```python
from build123d import *

# Parameters (mm, degrees)
SKETCH2_R = 12.85


with BuildPart() as part:
    # Sweep1: sweep along a path in Sketch1
    with BuildLine() as sweep1_path:  # in the path sketch's own coordinates; laid on its plane below (add() does not lay a ready-made edge on the line's plane)
        Line((301.307150881, 29.86530187), (131.307150881, 29.86530187))
        add(Edge.make_bspline(
            [(131.307150881, 29.86530187), (90.533603326, 8.116674685), (47, 8.116674685)],
            knots=[0, 0, 0, 1, 1, 1], degree=2))
        Line((47, 8.116674685), (0, 8.116674685))
    # Sketch2 → Sweep1 (sweep)
    with BuildSketch(Plane(origin=(301.307150881, 0, 0), x_dir=(0, 0, -1), z_dir=(1, 0, 0))):
        with Locations((29.86530187, 0)):
            Circle(SKETCH2_R)
    sweep1 = sweep(path=Plane(origin=(0, 0, 0), x_dir=(1, 0, 0), z_dir=(0, 1, 0)) * sweep1_path.line, transition=Transition.RIGHT)

    # Mirror1: Sweep1 across plane
    add(sweep1.mirror(Plane(origin=(0, 0, 0), x_dir=(0, 0, 1), z_dir=(1, 0, 0))))


solid = part.part
```
Source: CAD feature listing. Evaluate the final solid. Frame: model axes, mm. A direction names the side the tool comes from. Coordinates: 2 decimals unless noted, no trailing zeros. Loops run counter-clockwise (first coordinate to the right, second up) from the corner with the lowest first, then second, coordinate; pieces in that order, holes last. Notation, with made-up numbers: (-23.5, 11.25) - (26.5, 11.25) arc R10 cw to (26.5, 23.25) - close; hole circle Ø4 at (72, -7). An arc over 180 degrees is marked (long way). Answer as CSV lines item,"result".
1. Mould query, pull axis X, two halves, no side actions, for faces 1 (the cylindrical face through (-213.488, 4.922, -41.735)), 2 (the flat face through (-301.307, 0, -30)), 3 (the cylindrical face through (0.658, 4.922, -19.987)). Classes: released by +X, released by -X, zero draft, split by the parting line, or undercut.
Established:
face 1,"zero draft"
face 2,"released by -X"
face 3,"undercut"
2. Reachability of faces 4 (the flat face through (301.307, 0, -30)), 5 (the cylindrical face through (213.488, 4.922, -41.735)) from +Z, -Z, +X, -X, +Y, -Y: full face, straight path, thin tool, end or side. Return the list, or none.
Established:
face 4,"+Z, -Z, +X, +Y, -Y"
face 5,"+X"
3. Contact query for flat-ended pins moving along their axis: pin 1 (5 mm diameter, centred on x = 38.5, z = -19.5, fed in from +Y); pin 2 (10 mm diameter, centred on x = -78.5, y = -3.5, fed in from -Z); pin 3 (3 mm diameter, centred on x = -143, z = -18.5, fed in from +Y). Output: stop coordinate, or through.
Established:
pin 1,"stops at y = 9.28"
pin 2,"stops at z = -25.03"
pin 3,"stops at y = 8.23"
4. Ray query, line 1 (X direction, y = -4.25, z = -35.5); line 2 (Z direction, x = 4, y = -1.75); line 3 (Y direction, x = 73, z = -10.5). Return the intervals inside material, ascending.
Established:
line 1,"x = -301.31 to -115.38, 115.38 to 301.31"
line 2,"z = -20.85 to 4.61"
line 3,"y = -12.84 to 12.84"
5. Section A-A (x = 226). Return loops of the section in (y, z).
Established:
outline,"circle Ø25.7 at (0, -29.87)"
